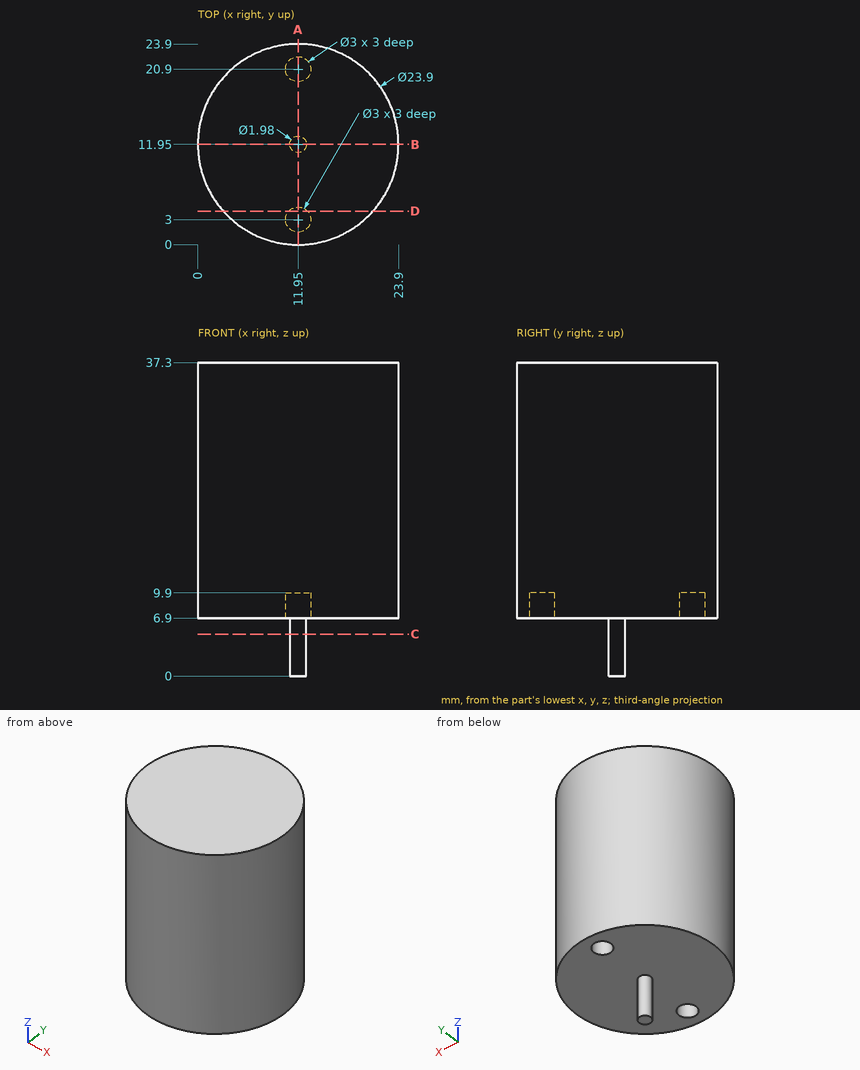
For this review, use the dimensioned drawing (mm, ordinates from the lowest corner) and the shaded views. Give positions to 0.01 mm unless a question says otherwise; leave off trailing zeros. Order: outer loops, then holes, each group sorted by start corner. A loop starts at its lowest first (then second) coordinate and runs counter-clockwise, first axis right, second up. Notation, with made-up numbers: (-21, 22.25) - (-9, 22.25) arc R24 ccw to (-9, 43.25) - close; hole circle Ø6 at (46, 14). An arc over 180 degrees is marked (long way). Use a Markdown table: item, result. Add a question column.
(1) Wall thickness on probe 1 along Y at (x, z) = (11.95, 8); probe 2 along Z at (x, y) = (2, 16); probe 3 along X at (y, z) = (2.5, 25.5): over which ranges is each line inside the solid? List them lowest first. Write a range as [from, to].
(2) Add section B-B on y = 11.95. Give the boundary of the cut face in (x, z).
(3) Clearance check with flat-ended pins moving along their axes: P1, Ø1.5, axis at x = 11.5, y = 21, coming from the -Z side; P2, Ø4, axis at x = 11.95, y = 20.9, coming from the -Z side; P3, Ø2, axis at x = 4.5, z = 21, coming from the +Y side. State where each tip first meets the part, or that it passes through.
(4) Add section D-D on y = 4. Give the boundary of the cut face in (x, z), then the cut area to 3 significant figures.
(5) Add section A-A on x = 11.95. Give the boundary of the cut face in (y, z), then the cut area to 3 significant figures.
(6) Add section C-C on z = 5. Give the boundary of the cut face in (x, y).
Report:
| question | item | result |
|---|---|---|
| 1 | probe 1 | y = [0, 1.5], [4.5, 19.4], [22.4, 23.9] |
| 1 | probe 2 | z = [6.9, 37.3] |
| 1 | probe 3 | x = [4.64, 19.26] |
| 2 | outline | (0, 6.9) - (10.96, 6.9) - (10.96, 0) - (12.94, 0) - (12.94, 6.9) - (23.9, 6.9) - (23.9, 37.3) - (0, 37.3) - close |
| 3 | P1 | stops at z = 9.9 |
| 3 | P2 | stops at z = 6.9 |
| 3 | P3 | stops at y = 22.01 |
| 4 | outline | (3.03, 6.9) - (10.83, 6.9) - (10.83, 9.9) - (13.07, 9.9) - (13.07, 6.9) - (20.87, 6.9) - (20.87, 37.3) - (3.03, 37.3) - close |
| 4 | area | 536 mm² |
| 5 | outline | (0, 6.9) - (1.5, 6.9) - (1.5, 9.9) - (4.5, 9.9) - (4.5, 6.9) - (10.96, 6.9) - (10.96, 0) - (12.94, 0) - (12.94, 6.9) - (19.4, 6.9) - (19.4, 9.9) - (22.4, 9.9) - (22.4, 6.9) - (23.9, 6.9) - (23.9, 37.3) - (0, 37.3) - close |
| 5 | area | 722 mm² |
| 6 | outline | circle Ø1.98 at (11.95, 11.95) |
